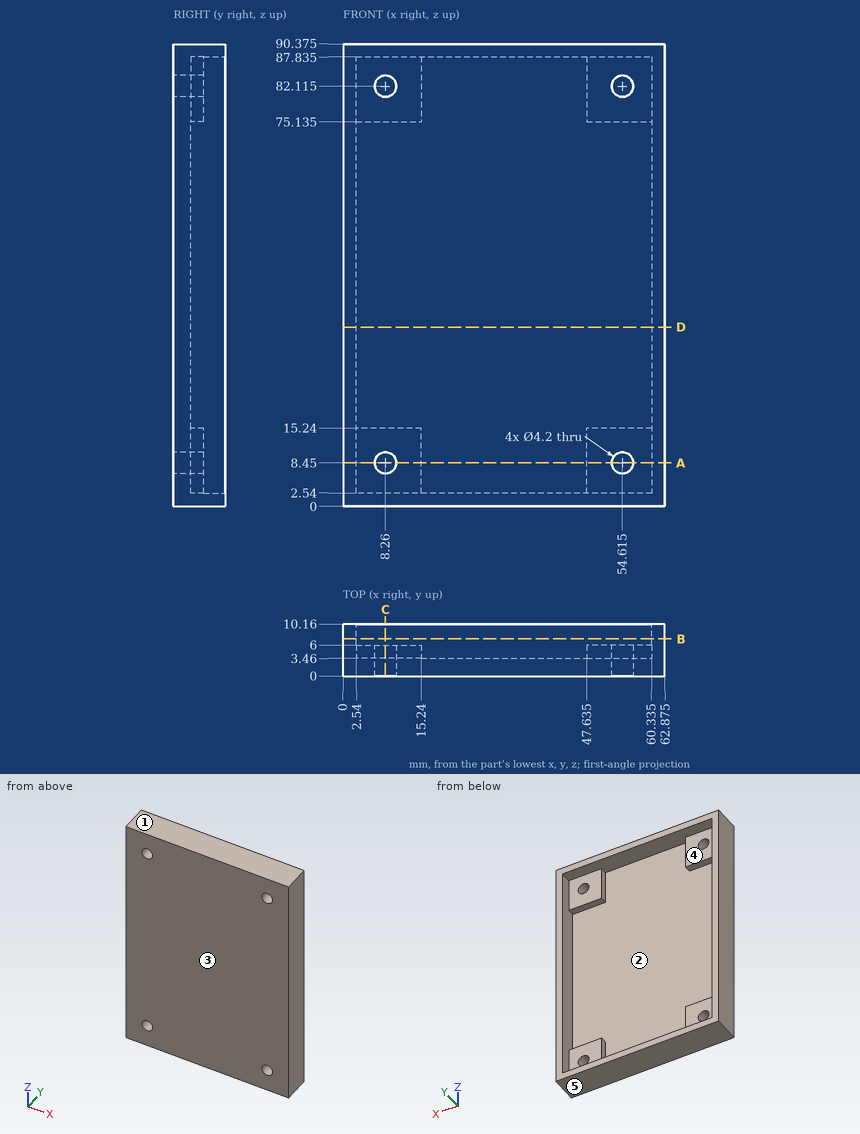
Study the drawing (mm; zero at the part's minimum x, y, z) and answer. A direction names the side the tool comes from. Round coordinates to 2 decimals unless told otherwise and drop trailing zeros. Write each loop counter-clockwise with the first axis right and the second up, starting at its lowest first coordinate (ties: lowest second). Pieces come first, ordered by that corner, then holes.
Q1. Straight lines are drawn through the part: line 1 (Z direction, x = 8.26, y = 2.4) (3 decimals); line 2 (Z direction, x = 8.26, y = 3.8) (3 decimals); line 3 (Z direction, x = 29.5, y = 9.75) (3 decimals). For each, find the intervals that lie inside material, in ascending order.
Values:
line 1: z = 0 to 6.35, 10.55 to 80.015, 84.215 to 90.375
line 2: z = 0 to 6.35, 10.55 to 15.24, 75.135 to 80.015, 84.215 to 90.375
line 3: z = 0 to 2.54, 87.835 to 90.375
Q2. Find section D-D on z = 35. Determine the outline of the cut face in (x, y) (3 decimals).
Values:
outline: (0, 0) - (62.875, 0) - (62.875, 10.16) - (60.335, 10.16) - (60.335, 3.46) - (2.54, 3.46) - (2.54, 10.16) - (0, 10.16) - close
Q3. Find section C-C on x = 8.26. Determine the outline of the cut face in (y, z) (3 decimals), and give its area (3 significant figures).
Values:
outline: (0, 0) - (10.16, 0) - (10.16, 2.54) - (6, 2.54) - (6, 6.35) - (0, 6.35) - close; (0, 10.55) - (6, 10.55) - (6, 15.24) - (3.46, 15.24) - (3.46, 75.135) - (6, 75.135) - (6, 80.015) - (0, 80.015) - close; (0, 84.215) - (6, 84.215) - (6, 87.835) - (10.16, 87.835) - (10.16, 90.375) - (0, 90.375) - close
area: 361 mm2
Q4. The mould has two halves that part along Z. Classify the marked faces 1, 2 and 3: released by +Z, released by -Z, zero draft, split by the parting line, or undercut.
Values:
face 1: released by +Z
face 2: undercut
face 3: zero draft
Q5. Find section A-A on z = 8.45. Determine the outline of the cut face in (x, y) (3 decimals).
Values:
outline: (0, 0) - (6.16, 0) - (6.16, 6) - (2.54, 6) - (2.54, 10.16) - (0, 10.16) - close; (10.36, 0) - (52.515, 0) - (52.515, 6) - (47.635, 6) - (47.635, 3.46) - (15.24, 3.46) - (15.24, 6) - (10.36, 6) - close; (56.715, 0) - (62.875, 0) - (62.875, 10.16) - (60.335, 10.16) - (60.335, 6) - (56.715, 6) - close
Q6. Flat-ended cylindrical pins translate along their axes: P1, Ø3, axis at x = 43.5, z = 61, coming from the +Y side; P2, Ø12, axis at x = 9, z = 21, coming from the +Y side. Find the tip coordinate at first contact, or state that the pin passes through.
Values:
P1: stops at y = 3.46
P2: stops at y = 6
Q7. A tool of negligible diameter and unlimited length cuts with its end or side. For the marked faces 4 and 5, from which of +Z, -Z, +X, -X, +Y, -Y can it reach the whole face along a straight path? Write none if from no direction.
Values:
face 4: +Y
face 5: -Z, +X, -X, +Y, -Y
Q8. Find section B-B on y = 7.25. Determine the outline of the cut face in (x, z) (3 decimals).
Values:
outline: (0, 0) - (62.875, 0) - (62.875, 90.375) - (0, 90.375) - close; hole (2.54, 2.54) - (60.335, 2.54) - (60.335, 87.835) - (2.54, 87.835) - close
